Model file for the job. Use its own axes, mm. A direction names the side the tool comes from. Coordinates: 2 decimals unless noted, no trailing zeros. Loops run counter-clockwise (first coordinate to the right, second up) from the corner with the lowest first, then second, coordinate; pieces in that order, holes last. Notation, with made-up numbers: (14, 48.5) - (45, 48.5) arc R15 ccw to (45, 66.5) - close; hole circle Ø2 at (79.5, 73). An arc over 180 degrees is marked (long way). Write each question's results on one line, items separated by ' | '. Start each with the question number.
```python
from build123d import *

# Parameters (mm, degrees)
BASES_W                     = 6
BASES_H                     = 6
BASE_DEPTH                  = 1
INSIDEWIREHOLDINGBODYS_R    = 3
INSIDEWIREHOLDINGBODY_DEPTH = 1.5
FRONTFACES_R                = 2.25
REARFACES_R                 = 2
HOLE_DEPTH                  = 9.185352857
HOLE_DEPTH_BACK             = 9.185352857
HOLES_R                     = 1.5
BASEFILLET_R                = 1


with BuildPart() as part:
    # BaseS → Base (new, symmetric)
    with BuildSketch(Plane(origin=(0, 0, 0), x_dir=(0, 0, -1), z_dir=(1, 0, 0))):
        Rectangle(BASES_W, BASES_H)
    extrude(amount=BASE_DEPTH, both=True)

    # InsideWireHoldingBodyS → InsideWireHoldingBody (add)
    with BuildSketch(Plane.ZY.offset(1)):
        Circle(INSIDEWIREHOLDINGBODYS_R)
    extrude(amount=INSIDEWIREHOLDINGBODY_DEPTH)

    # FrontFaceS → StrainReliefBody section 0
    with BuildSketch(Plane(origin=(1, 0, 0), x_dir=(0, 0, -1), z_dir=(1, 0, 0))):
        Circle(FRONTFACES_R)
    # RearFaceS → StrainReliefBody section 1
    with BuildSketch(Plane(origin=(7, 0, 0), x_dir=(0, 0, -1), z_dir=(1, 0, 0))):
        Circle(REARFACES_R)
    loft()

    # HoleS → Hole (cut, two sides: drawn at the far end of the back side and taken through both)
    with BuildSketch(Plane(origin=(0, 0, 0), x_dir=(0, 0, -1), z_dir=(1, 0, 0)).offset(-HOLE_DEPTH_BACK)):
        Circle(HOLES_R)
    extrude(amount=HOLE_DEPTH + HOLE_DEPTH_BACK, mode=Mode.SUBTRACT)

    # BaseFillet
    basefillet_edges = [part.edges().sort_by_distance(p)[0] for p in [
        (0, -3, -3),
        (0, -3, 3),
        (0, 3, 3),
        (0, 3, -3),
    ]]
    fillet(basefillet_edges, radius=BASEFILLET_R)


solid = part.part
```
Q1. Cut at A-A (y = 2.65). List the corners of the cut face in (x, z), and give its area (3 significant figures).
Q2. Drill centre lines: L1, parallel to Z at x = 0.25, y = 0; L2, parallel to Z at x = 2.25, y = 0. Where is each one in solid material? Low to high. Write a range as from..to.
Q3. Cut at D-D (x = 6). List the corners of the cut face in (y, z).
Q4. Pin check, flat tips, straight feed: pin 1 (1.5 mm diameter, centred on x = 5, z = 0, fed in from -Y); pin 2 (2.5 mm diameter, centred on y = 0, z = 0, fed in from +X). Stop position of each tip, or through.
Q5. Cut at C-C (y = -2.4). List the corners of the cut face in (x, z).
Q6. Which spindle directions (+Z, -Z, +X, -X, +Y, -Y) get a long thin tool onto all of the face, cutting with end or side? Do faces 1 (the flat face through (-1, 2.2, 2.3)), 2 (the flat face through (-1, -2.3, -2.3)), 3 (the flat face through (-1, -2.3, 2.3)), 4 (the flat face through (1, -2, 1.4)). Say none if no direction does.
Q7. Cut at B-B (x = 2). List the corners of the cut face in (y, z), and give its area (3 significant figures).
Check result:
1) outline: (-2.5, -1.41) - (-1, -1.41) - (-1, -2.76) - (1, -2.76) - (1, 2.76) - (-1, 2.76) - (-1, 1.41) - (-2.5, 1.41) - close | area: 15.3 mm²
2) L1: -3..-1.5, 1.5..3 | L2: -2.2..-1.5, 1.5..2.2
3) outline: circle Ø4.08 at (0, 0); hole circle Ø3 at (0, 0)
4) pin 1: y = -2.11 | pin 2: through
5) outline: (-2.5, -1.8) - (-1, -1.8) - (-1, -2.92) - (1, -2.92) - (1, 2.92) - (-1, 2.92) - (-1, 1.8) - (-2.5, 1.8) - close
6) face 1: +Z, -X, +Y | face 2: -Z, -X, -Y | face 3: +Z, -X, -Y | face 4: +X
7) outline: circle Ø4.42 at (0, 0); hole circle Ø3 at (0, 0) | area: 8.25 mm²
